Build history of the part. All positions in model axes, mm. A direction names the side the tool comes from. Give positions to 0.01 mm unless a question says otherwise; leave off trailing zeros. Write each loop counter-clockwise with the first axis right and the second up, starting at its lowest first coordinate (ties: lowest second). Pieces come first, ordered by that corner, then holes. Notation, with made-up numbers: (46, 39) - (81, 39) arc R22 ccw to (81, 72) - close; hole circle Ø9 at (34, 67.5). An arc over 180 degrees is marked (long way). Use one line per item in the form item = value. Start each with the question number.
from build123d import *

# Parameters (mm, degrees)
BASES_R                     = 6.4
BASE_DEPTH                  = 5.6
TOPBORES_R                  = 1.4
TOP_BORE_DEPTH              = 11.643307757
HORN_HALF_DEPTH             = 2.5
HORNATTACHS_R               = 0.75
HORN_ATTACH_DEPTH           = 21.999047597
HA_LP_COUNT                 = 4
HA_LP_PITCH                 = 3
HORN_BODIES_COPY_1_SKETCH_R = 0.75
HORN_BODIES_COPY_1_DEPTH    = 21.999047597
HORN_BODIES_COPY_2_SKETCH_R = 0.75
HORN_BODIES_COPY_2_DEPTH    = 21.999047597
HORN_BODIES_COPY_3_SKETCH_R = 0.75
HORN_BODIES_COPY_3_DEPTH    = 21.999047597
TOOTH_DEPTH                 = 3
TOOTH_CP_COUNT              = 26
BOTTOMBORES_R               = 2.6
BOTTOM_BORE_DEPTH           = 3
HOLDINGSHAFTS_R             = 6.4
HOLDINGSHAFTS_R_2           = 4.25
HOLDING_SHAFT_DEPTH         = 3.1
RIB_DEPTH                   = 0.5
RIB_CP_COUNT                = 4
TOPCUTS_R                   = 4.45
TOP_CUT_DEPTH               = 1
TOPPOCKETCYLINDERS_R        = 3.45
TOPPOCKETCYLINDERS_R_2      = 2.95
TOP_POCKET_CYLINDER_DEPTH   = 1.35


with BuildPart() as part:
    # BaseS → BASE (new body)
    with BuildSketch(Plane(origin=(0, 0, 0), x_dir=(1, 0, 0), z_dir=(0, 1, 0))):
        with Locations(Location((0, 0, 0), (0, 0, 270))):
            Circle(BASES_R)
    extrude(amount=BASE_DEPTH)

    # TopBoreS → TOP BORE (cut, through all)
    with BuildSketch(Plane(origin=(0, 5.6, 0), x_dir=(1, 0, 0), z_dir=(0, 1, 0))):
        with Locations(Location((0, 0, 0), (0, 0, 270))):
            Circle(TOPBORES_R)
    extrude(amount=-TOP_BORE_DEPTH, mode=Mode.SUBTRACT)

    # HornHalfS → HORN HALF (add)
    with BuildSketch(Plane(origin=(0, 5.6, 0), x_dir=(1, 0, 0), z_dir=(0, 1, 0))):
        with BuildLine():
            Line((-2.609740545, 17.010167671), (-4.878700663, 4.142255405))
            ThreePointArc((-4.878700663, 4.142255405), (0, 6.4), (4.878700663, 4.142255405))
            Line((4.878700663, 4.142255405), (2.609740545, 17.010167671))
            ThreePointArc((2.609740545, 17.010167671), (0, 19.2), (-2.609740545, 17.010167671))
        make_face()
    horn_half = extrude(amount=-HORN_HALF_DEPTH)

    # HornAttachS → HORN ATTACH (cut, through all)
    with BuildSketch(Plane(origin=(0, 5.6, 0), x_dir=(1, 0, 0), z_dir=(0, 1, 0))):
        with Locations(Location((0, 16.2, 0), (0, 0, 270))):
            Circle(HORNATTACHS_R)
    horn_attach = extrude(amount=-HORN_ATTACH_DEPTH, mode=Mode.SUBTRACT)

    # HA LP: HORN ATTACH ×4
    with Locations(*[(0, 0, i * HA_LP_PITCH) for i in range(1, HA_LP_COUNT)]):
        add(horn_attach, mode=Mode.SUBTRACT)

    # HORN BODIES: HORN HALF, HORN ATTACH across plane
    add(horn_half.mirror(Plane.XY))
    add(horn_attach.mirror(Plane.XY), mode=Mode.SUBTRACT)

    # HORN BODIES copy 1 sketch → HORN BODIES copy 1 (cut, through all)
    with BuildSketch(Plane(origin=(0, 5.6, -3), x_dir=(1, 0, 0), z_dir=(0, 1, 0))):
        with Locations((0, -16.2)):
            Circle(HORN_BODIES_COPY_1_SKETCH_R)
    extrude(amount=-HORN_BODIES_COPY_1_DEPTH, mode=Mode.SUBTRACT)

    # HORN BODIES copy 2 sketch → HORN BODIES copy 2 (cut, through all)
    with BuildSketch(Plane(origin=(0, 5.6, -6), x_dir=(1, 0, 0), z_dir=(0, 1, 0))):
        with Locations((0, -16.2)):
            Circle(HORN_BODIES_COPY_2_SKETCH_R)
    extrude(amount=-HORN_BODIES_COPY_2_DEPTH, mode=Mode.SUBTRACT)

    # HORN BODIES copy 3 sketch → HORN BODIES copy 3 (cut, through all)
    with BuildSketch(Plane(origin=(0, 5.6, -9), x_dir=(1, 0, 0), z_dir=(0, 1, 0))):
        with Locations((0, -16.2)):
            Circle(HORN_BODIES_COPY_3_SKETCH_R)
    extrude(amount=-HORN_BODIES_COPY_3_DEPTH, mode=Mode.SUBTRACT)

    # ToothS → TOOTH (cut)
    with BuildSketch(Plane.XZ):
        with BuildLine():
            Line((0, -2.9), (0.262912611, -2.586672952))
            ThreePointArc((0.262912611, -2.586672952), (0, -2.6), (-0.262912611, -2.586672952))
            Line((-0.262912611, -2.586672952), (0, -2.9))
        make_face()
    tooth = extrude(amount=-TOOTH_DEPTH, mode=Mode.SUBTRACT)

    # TOOTH CP: TOOTH ×26 about axis
    tooth_cp_axis = Axis((0, 0, 0), (0, 1, 0))
    for i in range(1, TOOTH_CP_COUNT):
        add(tooth.rotate(tooth_cp_axis, i * 360 / TOOTH_CP_COUNT), mode=Mode.SUBTRACT)

    # BottomBoreS → BOTTOM BORE (cut)
    with BuildSketch(Plane(origin=(0, 0, 0), x_dir=(-1, 0, 0), z_dir=(0, -1, 0))):
        Circle(BOTTOMBORES_R)
    extrude(amount=-BOTTOM_BORE_DEPTH, mode=Mode.SUBTRACT)

    # HoldingShaftS → HOLDING SHAFT (cut)
    with BuildSketch(Plane.XZ):
        Circle(HOLDINGSHAFTS_R)
        with Locations(Location((0, 0, 0), (0, 0, 270))):
            Circle(HOLDINGSHAFTS_R_2, mode=Mode.SUBTRACT)
    extrude(amount=-HOLDING_SHAFT_DEPTH, mode=Mode.SUBTRACT)

    # RibS → RIB (add, symmetric)
    with BuildSketch(Plane.XY):
        Polygon((4.21, 1.2), (5.804289299, 3.1), (4.21, 3.1), (4.16, 3.1), (4.16, 1.2), align=None)
    rib = extrude(amount=RIB_DEPTH, both=True)

    # RIB CP: RIB ×4 about axis
    rib_cp_axis = Axis((0, 0, 0), (0, 1, 0))
    for i in range(1, RIB_CP_COUNT):
        add(rib.rotate(rib_cp_axis, i * 360 / RIB_CP_COUNT))

    # TopCutS → TOP CUT (cut)
    with BuildSketch(Plane(origin=(0, 5.6, 0), x_dir=(1, 0, 0), z_dir=(0, 1, 0))):
        with Locations(Location((0, 0, 0), (0, 0, 270))):
            Circle(TOPCUTS_R)
    extrude(amount=-TOP_CUT_DEPTH, mode=Mode.SUBTRACT)

    # TopPocketCylinderS → TOP POCKET CYLINDER (add)
    with BuildSketch(Plane(origin=(0, 4.6, 0), x_dir=(1, 0, 0), z_dir=(0, 1, 0))):
        with Locations(Location((0, 0, 0), (0, 0, 270))):
            Circle(TOPPOCKETCYLINDERS_R)
        with Locations(Location((0, 0, 0), (0, 0, 270))):
            Circle(TOPPOCKETCYLINDERS_R_2, mode=Mode.SUBTRACT)
    extrude(amount=TOP_POCKET_CYLINDER_DEPTH)


solid = part.part
(1) Cut at B-B, the plane x = -5.25. Give the cut face in (y, z).
(2) Pin check, flat tips, straight feed: pin 1 Ø1 at (x, y) = (-1.5, 2.5) entering from +Z; pin 2 Ø1.4 at (x, z) = (0, 10.2) entering from -Y; pin 3 Ø0.5 at (x, y) = (-5, 2) entering from -Z; pin 4 Ø4 at (x, z) = (2.5, 10.5) entering from +Y. Stop position of each tip, or through.
(3) Which spindle directions (+Z, -Z, +X, -X, +Y, -Y) get a long thin tool onto all of the face, cutting with end or side? Do faces 5 (the flat face through (-0.5, 2.4, 4.8)), 6 (the cylindrical face through (-2.88, 5.27, -0.64)), 7 (the cylindrical face through (6.4, 4.3, 0.1)), 8 (the flat face through (0.5, 2.4, -4.8)). Say none if no direction does.
(4) Two-plate mould, pull along X, no slides. Class faces 1 (the flat face through (1, 5.95, 3)), 2 (the cylindrical face through (0.03, 4.37, -16.95)), 3 (the cylindrical face through (0.1, 4.4, 19.2)), 4 (the flat face through (3.76, 4.37, -10.49)): +X half, -X half, draft (parallel to the pull), parting line (faces both ways), or undercut.
(5) Wall check: line 1 (Y direction, x = -3, z = 12); line 2 (X direction, y = 0.85, z = -1); line 3 (X direction, y = 5.55, z = 3.5). Give the ranges that are in metal, low to high. Write a range as from..to.
(6) Cut at C-C, the plane z = 16.2. Give the cut face in (x, y), then the cut area to 3 significant figures.
(7) Cut at A-A, the plane z = -10.2. Give the cut face in (x, y), then the cut area to 3 significant figures.
(8) Cut at D-D, the plane z = -14.5. Give the cut face in (x, y).
Solution:
q1.outline = (2.44, -0.5) - (3.1, -0.5) - (3.1, -3.66) - (5.6, -3.66) - (5.6, 3.66) - (3.1, 3.66) - (3.1, 0.5) - (2.44, 0.5) - close
q2.pin_1 = 4.13
q2.pin_2 = through
q2.pin_3 = -0.5
q2.pin_4 = 5.6
q3.face_5 = +Z, -X, -Y
q3.face_6 = +Y
q3.face_7 = +X, +Y, -Y
q3.face_8 = -Z, +X, -Y
q4.face_1 = draft
q4.face_2 = undercut
q4.face_3 = parting line
q4.face_4 = +X half
q5.line_1 = 3.1..5.6
q5.line_2 = -4.13..-2.7, 2.7..4.13
q5.line_3 = -5.36..-2.75, 2.75..5.36
q6.outline = (-2.75, 3.1) - (-0.75, 3.1) - (-0.75, 5.6) - (-2.75, 5.6) - close; (0.75, 3.1) - (2.75, 3.1) - (2.75, 5.6) - (0.75, 5.6) - close
q6.area = 10.0 mm2
q7.outline = (-3.81, 3.1) - (-0.75, 3.1) - (-0.75, 5.6) - (-3.81, 5.6) - close; (0.75, 3.1) - (3.81, 3.1) - (3.81, 5.6) - (0.75, 5.6) - close
q7.area = 15.3 mm2
q8.outline = (-3.05, 3.1) - (3.05, 3.1) - (3.05, 5.6) - (-3.05, 5.6) - close
